Model file for the job. Use its own axes, mm. Face numbers are marked on the shaded views. Give positions to 0.01 mm unless a question says otherwise; leave off trailing zeros. Write each loop counter-clockwise with the first axis right and the second up, starting at its lowest first coordinate (ties: lowest second). Pieces come first, ordered by that corner, then holes.
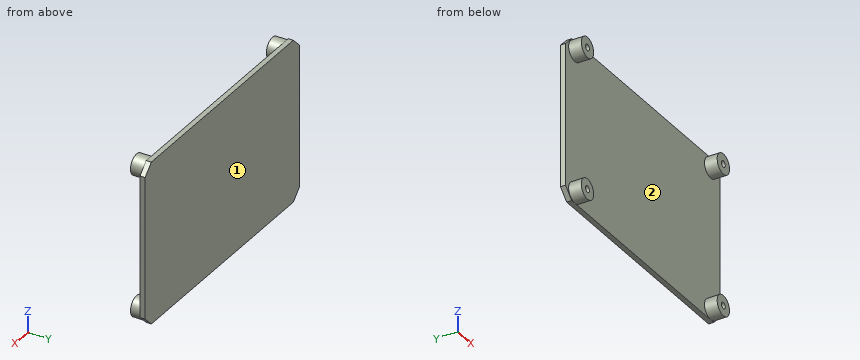
```python
from build123d import *

# Parameters (mm, degrees)
SHADE_PLATE_DEPTH = 2
SKETCH2_R         = 4
POSTS_DEPTH       = 5.1
SKETCH3_R         = 1.25
POST_PILOTS_DEPTH = 6.5


with BuildPart() as part:
    # Sketch1 → Shade Plate (new body)
    with BuildSketch(Plane(origin=(0, 17.4, 0), x_dir=(1, 0, 0), z_dir=(0, 1, 0))):
        Polygon((-46, -84), (46, -84), (50, -80), (50, -24), (46, -20), (-46, -20), (-50, -24), (-50, -80), align=None)
    extrude(amount=SHADE_PLATE_DEPTH)

    # Sketch2 → Posts (add)
    with BuildSketch(Plane(origin=(0, 12.4, 0), x_dir=(1, 0, 0), z_dir=(0, 1, 0))):
        with Locations(Location((-44, -24, 0), (0, 0, 90))):
            Circle(SKETCH2_R)
        with Locations(Location((-44, -80, 0), (0, 0, 270))):
            Circle(SKETCH2_R)
        with Locations(Location((44, -24, 0), (0, 0, 90))):
            Circle(SKETCH2_R)
        with Locations(Location((44, -80, 0), (0, 0, 270))):
            Circle(SKETCH2_R)
    extrude(amount=POSTS_DEPTH)

    # Sketch3 → Post Pilots (cut)
    with BuildSketch(Plane(origin=(0, 11.9, 0), x_dir=(1, 0, 0), z_dir=(0, 1, 0))):
        with Locations(Location((-44, -24, 0), (0, 0, 270))):
            Circle(SKETCH3_R)
        with Locations(Location((-44, -80, 0), (0, 0, 270))):
            Circle(SKETCH3_R)
        with Locations(Location((44, -24, 0), (0, 0, 270))):
            Circle(SKETCH3_R)
        with Locations(Location((44, -80, 0), (0, 0, 270))):
            Circle(SKETCH3_R)
    extrude(amount=POST_PILOTS_DEPTH, mode=Mode.SUBTRACT)


solid = part.part
```
1. Slice it at C-C, the plane x = 14.5. Write the cut outline in (y, z), and give its area (3 significant figures).
Calculated:
outline: (17.4, 20) - (19.4, 20) - (19.4, 84) - (17.4, 84) - close
area: 128 mm2
2. Slice it at A-A, the plane y = 14.5. Write the cut outline in (x, z), and give its area (3 significant figures).
Calculated:
outline: circle Ø8 at (-44, 24); circle Ø8 at (-44, 80); circle Ø8 at (44, 24); circle Ø8 at (44, 80); hole circle Ø2.5 at (-44, 24); hole circle Ø2.5 at (-44, 80); hole circle Ø2.5 at (44, 24); hole circle Ø2.5 at (44, 80)
area: 181 mm2
3. Slice it at B-B, the plane z = 67.5. Write the cut outline in (x, y).
Calculated:
outline: (-50, 17.4) - (50, 17.4) - (50, 19.4) - (-50, 19.4) - close
4. Pin check, flat tips, straight feed: P1, Ø1, axis at x = 15.5, z = 30.5, coming from the -Y side; P2, Ø0.8, axis at x = 44.5, z = 24.5, coming from the -Y side. Stop position of each tip, or through.
Calculated:
P1: stops at y = 17.4
P2: stops at y = 18.4
5. Probe probe 1 along X at (y, z) = (14.4, 80); probe 2 along Z at (x, y) = (-44, 15.4); probe 3 along X at (y, z) = (17.5, 23). List the from-to ranges inside material, lowest first.
Calculated:
probe 1: x = -48 to -45.25, -42.75 to -40, 40 to 42.75, 45.25 to 48
probe 2: z = 20 to 22.75, 25.25 to 28, 76 to 78.75, 81.25 to 84
probe 3: x = -49 to -44.75, -43.25 to 43.25, 44.75 to 49
6. Pull direction X, two halves, no side cores. Call the marked faces 1 and 2: +X half, -X half, draft (parallel to the pull), parting line (faces both ways), or undercut.
Calculated:
face 1: draft
face 2: undercut
